Verification items for the finished model (mm, model axes). A direction names the side the tool comes from. Give positions to 0.01 mm unless a question says otherwise; leave off trailing zeros. Loops run counter-clockwise (first coordinate to the right, second up) from the corner with the lowest first, then second, coordinate; pieces in that order, holes last. Notation, with made-up numbers: (-33, 54) - (-1, 54) arc R16 ccw to (-1, 58) - close; hole circle Ø6 at (73.25, 58.5). An arc over 180 degrees is marked (long way). One line per item, written item: value. Start each with the question number.
1. Gauge pin test, flat ends, axial feed: pin 1 (1 mm diameter, centred on y = -89, z = 1.5, fed in from +X); pin 2 (2.5 mm diameter, centred on x = -134.52, y = 28.25, fed in from +Z). Record the tip position at first contact, or that the pin passes through.
2. Sectioned sample at A-A (x = -24). Record the cut outline in (y, z).
3. Mould release check, pull along X, two halves, no side actions. Record for faces 1 (the cylindrical face through (-125.656, 64.409, 1.479)), 2 (the cylindrical face through (-23.61, -116.667, 1.479)), 3 (the flat face through (-35.4, 10.744, 1.479)): pulls with the +X half, pulls with the -X half, needs draft (parallel to the pull), parting line crosses it, or undercut.
4. Sectioned sample at B-B (y = 80). Record the cut outline in (x, z).
5. Access from +Z, -Z, +X, -X, +Y, -Y to the whole of each face (thin tool, end or side, straight path). Record for faces 4 (the flat face through (3.669, -11.586, 1.479)), 5 (the flat face through (3, 3, 3)).
6. Sectioned sample at C-C (z = 2.5). Count the separate pieces of the cut face and the enclosed holes in it, plus the area to 3 significant figures.
7. Scan lines: L1, parallel to Y at x = -8, z = 2.05; L2, parallel to X at y = -3.5, z = 0.7; L3, parallel to X at y = -7, z = 1.15. Record each from-to range of solid material in increasing order. Write a range as [from, to].
from build123d import *

# Parameters (mm, degrees)
SKETCH1_R           = 1.475
SKETCH1_R_2         = 8
BOSS_EXTRUDE1_DEPTH = 3
FILLET1_START       = -1
FILLET1_DEPTH       = 5
SKETCH2_R           = 1.475
CUT_EXTRUDE1_DEPTH  = 186.540999332


with BuildPart() as part:
    # Sketch1 → Boss-Extrude1 (new body)
    with BuildSketch(Plane.XY):
        with BuildLine():
            Line((0.526015848, 103.328982943), (-45.247486844, 103.328982943))
            Line((-45.247486844, 103.328982943), (-45.247486844, 121.128982943))
            ThreePointArc((-45.247486844, 121.128982943), (-126.28610555, 63.330323318), (-135.821903737, -35.750508981))
            Line((-135.821903737, -35.750508981), (-120.406651549, -26.850508981))
            Line((-120.406651549, -26.850508981), (-97.519900204, -66.491525133))
            Line((-97.519900204, -66.491525133), (-112.935152391, -75.391525133))
            ThreePointArc((-112.935152391, -75.391525133), (-22.360735498, -116.673697807), (68.213681395, -75.391525133))
            Line((68.213681395, -75.391525133), (52.798429207, -66.491525133))
            Line((52.798429207, -66.491525133), (75.685180553, -26.850508981))
            Line((75.685180553, -26.850508981), (91.100432741, -35.750508981))
            ThreePointArc((91.100432741, -35.750508981), (81.564634554, 63.330323318), (0.526015848, 121.128982943))
            Line((0.526015848, 121.128982943), (0.526015848, 103.328982943))
        make_face()
        with Locations((67.384177861, -31.228267397)):
            Circle(SKETCH1_R, mode=Mode.SUBTRACT)
        with Locations((52.439177861, -57.113766716)):
            Circle(SKETCH1_R, mode=Mode.SUBTRACT)
        with Locations((-97.160648858, -57.113766716)):
            Circle(SKETCH1_R, mode=Mode.SUBTRACT)
        with Locations((-56.860735498, -106.258884513)):
            Circle(SKETCH1_R, mode=Mode.SUBTRACT)
        with Locations((-112.105648858, -31.228267397)):
            Circle(SKETCH1_R, mode=Mode.SUBTRACT)
        with Locations((-91.269077643, -19.198267397)):
            Circle(SKETCH1_R, mode=Mode.SUBTRACT)
        with Locations((-76.324077643, -45.083766716)):
            Circle(SKETCH1_R, mode=Mode.SUBTRACT)
        with Locations((-56.860735498, -52.258884513)):
            Circle(SKETCH1_R, mode=Mode.SUBTRACT)
        with Locations((12.139264502, -106.258884513)):
            Circle(SKETCH1_R, mode=Mode.SUBTRACT)
        with Locations((-12.112024192, -34.919728363)):
            Circle(SKETCH1_R, mode=Mode.SUBTRACT)
        with Locations((12.139264502, -52.258884513)):
            Circle(SKETCH1_R, mode=Mode.SUBTRACT)
        with Locations((31.602606646, -45.083766716)):
            Circle(SKETCH1_R, mode=Mode.SUBTRACT)
        with BuildLine():
            ThreePointArc((0.120026615, -17.733194883), (-1.094386102, -18.665046536), (-2.612024192, -18.465245691))
            ThreePointArc((-2.612024192, -18.465245691), (-3.543875845, -17.250832974), (-3.344075, -15.733194883))
            Line((-3.344075, -15.733194883), (3.655925, -3.60883923))
            ThreePointArc((3.655925, -3.60883923), (4.870337718, -2.676987578), (6.387975808, -2.876788423))
            ThreePointArc((6.387975808, -2.876788423), (7.31982746, -4.09120114), (7.120026615, -5.60883923))
            Line((7.120026615, -5.60883923), (0.120026615, -17.733194883))
        make_face(mode=Mode.SUBTRACT)
        with Locations((46.547606646, -19.198267397)):
            Circle(SKETCH1_R, mode=Mode.SUBTRACT)
        with Locations((-87.751240857, 1.245040241)):
            Circle(SKETCH1_R, mode=Mode.SUBTRACT)
        with Locations((-134.516612662, 28.245040241)):
            Circle(SKETCH1_R, mode=Mode.SUBTRACT)
        with Locations((-68.733802457, 7.008474867)):
            Circle(SKETCH1_R, mode=Mode.SUBTRACT)
        with BuildLine():
            Line((-28.38701494, 14.89116077), (-35.38701494, 2.766805117))
            ThreePointArc((-35.38701494, 2.766805117), (-38.119065747, 2.034754309), (-38.851116555, 4.766805117))
            Line((-38.851116555, 4.766805117), (-31.851116555, 16.89116077))
            ThreePointArc((-31.851116555, 16.89116077), (-29.119065747, 17.623211577), (-28.38701494, 14.89116077))
        make_face(mode=Mode.SUBTRACT)
        with Locations((-48.733802457, 41.649491019)):
            Circle(SKETCH1_R, mode=Mode.SUBTRACT)
        with Locations((-100.016612662, 88.000793102)):
            Circle(SKETCH1_R, mode=Mode.SUBTRACT)
        with Locations((-53.251240857, 61.000793102)):
            Circle(SKETCH1_R, mode=Mode.SUBTRACT)
        with Locations((-37.305735498, 74.268982943)):
            Circle(SKETCH1_R, mode=Mode.SUBTRACT)
        with Locations((-37.305735498, 98.328982943)):
            Circle(SKETCH1_R, mode=Mode.SUBTRACT)
        with Locations((-22.360735498, 3.328982943)):
            Circle(SKETCH1_R_2, mode=Mode.SUBTRACT)
        with Locations((15.887975808, 13.577694249)):
            Circle(SKETCH1_R, mode=Mode.SUBTRACT)
        with Locations((43.029769861, 1.245040241)):
            Circle(SKETCH1_R, mode=Mode.SUBTRACT)
        with Locations((89.795141666, 28.245040241)):
            Circle(SKETCH1_R, mode=Mode.SUBTRACT)
        with Locations((8.529769861, 61.000793102)):
            Circle(SKETCH1_R, mode=Mode.SUBTRACT)
        with Locations((-7.415735498, 74.268982943)):
            Circle(SKETCH1_R, mode=Mode.SUBTRACT)
        with Locations((-7.415735498, 98.328982943)):
            Circle(SKETCH1_R, mode=Mode.SUBTRACT)
        with Locations((55.295141666, 88.000793102)):
            Circle(SKETCH1_R, mode=Mode.SUBTRACT)
    extrude(amount=BOSS_EXTRUDE1_DEPTH)

    # Fillet1: read off the stored shape, not the designer's step
    # Fillet1 outline → Fillet1 (cut)
    with BuildSketch(Plane.XY.offset(FILLET1_START)):
        with BuildLine():
            ThreePointArc((-45.247486844, 121.128982943), (-51.788195876, 119.667574833), (-58.237118653, 117.843298724))
            add(Edge.make_bspline(
                [(-58.237118653, 117.843298724), (-56.095583294, 118.514223949), (-53.982026531, 119.121408989), (-49.353840332, 119.42067321), (-46.388701083, 117.326670501), (-45.247486844, 112.620410582), (-45.247486844, 110.460531419), (-45.247486844, 108.300652255)],
                knots=[0, 0, 0, 0, 0, 0, 0.5, 0.5, 1, 1, 1, 1, 1, 1], degree=5))
            Line((-45.247486844, 108.300652255), (-45.247486844, 121.128982943))
        make_face()
        with BuildLine():
            add(Edge.make_bspline(
                [(-124.712243473, -29.336343637), (-126.582753698, -30.416283219), (-128.453263923, -31.496222801), (-133.099611688, -32.861032238), (-136.395640855, -31.340147677), (-138.450563536, -27.182388745), (-138.981504249, -25.048402376), (-139.471233639, -22.858315739)],
                knots=[0, 0, 0, 0, 0, 0, 0.5, 0.5, 1, 1, 1, 1, 1, 1], degree=5))
            ThreePointArc((-139.471233639, -22.858315739), (-137.826641704, -29.355384745), (-135.821903737, -35.750508981))
            Line((-135.821903737, -35.750508981), (-124.712243473, -29.336343637))
        make_face()
        with BuildLine():
            ThreePointArc((91.100432741, -35.750508981), (93.105170708, -29.355384745), (94.749762643, -22.858315739))
            add(Edge.make_bspline(
                [(94.749762643, -22.858315739), (94.260033253, -25.048402376), (93.72909254, -27.182388745), (91.674169859, -31.340147677), (88.378140692, -32.861032238), (83.731792926, -31.496222801), (81.861282701, -30.416283219), (79.990772476, -29.336343637)],
                knots=[0, 0, 0, 0, 0, 0, 0.5, 0.5, 1, 1, 1, 1, 1, 1], degree=5))
            Line((79.990772476, -29.336343637), (91.100432741, -35.750508981))
        make_face()
        with BuildLine():
            Line((0.526015848, 121.128982943), (0.526015848, 108.300652255))
            add(Edge.make_bspline(
                [(0.526015848, 108.300652255), (0.526015848, 110.460531419), (0.526015848, 112.620410582), (1.667230086, 117.326670501), (4.632369336, 119.42067321), (9.260555535, 119.121408989), (11.374112298, 118.514223949), (13.515647657, 117.843298724)],
                knots=[0, 0, 0, 0, 0, 0, 0.5, 0.5, 1, 1, 1, 1, 1, 1], degree=5))
            ThreePointArc((13.515647657, 117.843298724), (7.06672488, 119.667574833), (0.526015848, 121.128982943))
        make_face()
        with BuildLine():
            ThreePointArc((-112.935152391, -75.391525133), (-108.399181326, -80.325241258), (-103.594850484, -84.998034156))
            add(Edge.make_bspline(
                [(-103.594850484, -84.998034156), (-105.246656452, -83.478872744), (-106.829272503, -81.952071414), (-109.402536021, -78.093576704), (-109.071646103, -74.478689433), (-105.566512577, -71.137238952), (-103.696002352, -70.05729937), (-101.825492127, -68.977359788)],
                knots=[0, 0, 0, 0, 0, 0, 0.5, 0.5, 1, 1, 1, 1, 1, 1], degree=5))
            Line((-101.825492127, -68.977359788), (-112.935152391, -75.391525133))
        make_face()
        with BuildLine():
            Line((68.213681395, -75.391525133), (57.104021131, -68.977359788))
            add(Edge.make_bspline(
                [(57.104021131, -68.977359788), (58.974531355, -70.05729937), (60.84504158, -71.137238952), (64.350175107, -74.478689433), (64.681065025, -78.093576704), (62.107801507, -81.952071414), (60.525185456, -83.478872744), (58.873379488, -84.998034156)],
                knots=[0, 0, 0, 0, 0, 0, 0.5, 0.5, 1, 1, 1, 1, 1, 1], degree=5))
            ThreePointArc((58.873379488, -84.998034156), (63.67771033, -80.325241258), (68.213681395, -75.391525133))
        make_face()
    extrude(amount=FILLET1_DEPTH, mode=Mode.SUBTRACT)

    # Sketch2 → Cut-Extrude1 (cut, through all)
    with BuildSketch(Plane.XY.offset(3)):
        with Locations((7.020831752, 113.07197549)):
            Circle(SKETCH2_R)
        with Locations((-51.742302749, 113.07197549)):
            Circle(SKETCH2_R)
        with Locations((-79.127551915, 101.737973696)):
            Circle(SKETCH2_R)
        with Locations((34.406080919, 101.737973696)):
            Circle(SKETCH2_R)
        with Locations((-0.147120048, 86.298982943)):
            Circle(SKETCH2_R)
        with Locations((-44.574350948, 86.298982943)):
            Circle(SKETCH2_R)
        with Locations((91.247358663, 3.285992676)):
            Circle(SKETCH2_R)
        with Locations((87.37026756, -26.097329688)):
            Circle(SKETCH2_R)
        with Locations((60.600199979, -18.918461767)):
            Circle(SKETCH2_R)
        with Locations((38.386584529, -57.393572347)):
            Circle(SKETCH2_R)
        with Locations((34.480542246, -95.037017543)):
            Circle(SKETCH2_R)
        with Locations((57.988700309, -76.987696972)):
            Circle(SKETCH2_R)
        with Locations((-79.202013242, -95.037017543)):
            Circle(SKETCH2_R)
        with Locations((-102.710171305, -76.987696972)):
            Circle(SKETCH2_R)
        with Locations((-83.108055525, -57.393572347)):
            Circle(SKETCH2_R)
        with Locations((-132.091738556, -26.097329688)):
            Circle(SKETCH2_R)
        with Locations((-105.321670975, -18.918461767)):
            Circle(SKETCH2_R)
        with Locations((-135.96882966, 3.285992676)):
            Circle(SKETCH2_R)
    extrude(amount=-CUT_EXTRUDE1_DEPTH, mode=Mode.SUBTRACT)


solid = part.part
Results are:
1. pin 1: stops at x = 54.89
1. pin 2: passes through
2. outline: (-116.66, 0) - (-4.5, 0) - (-4.5, 3) - (-116.66, 3) - close; (11.16, 0) - (103.33, 0) - (103.33, 3) - (11.16, 3) - close
3. face 1: pulls with the -X half
3. face 2: parting line crosses it
3. face 3: undercut
4. outline: (-114.68, 0) - (69.96, 0) - (69.96, 3) - (-114.68, 3) - close
5. face 4: +Z, -Z
5. face 5: +Z, +X, -X, +Y, -Y
6. separate pieces: 1
6. enclosed holes: 49
6. area: 41,800 mm^2
7. L1: y = [-115.81, 72.91], [75.62, 96.97], [99.68, 103.33]
7. L2: x = [-142.17, -26.53], [-18.19, 3.72], [7.05, 97.45]
7. L3: x = [-141.92, 1.7], [6.32, 97.2]
